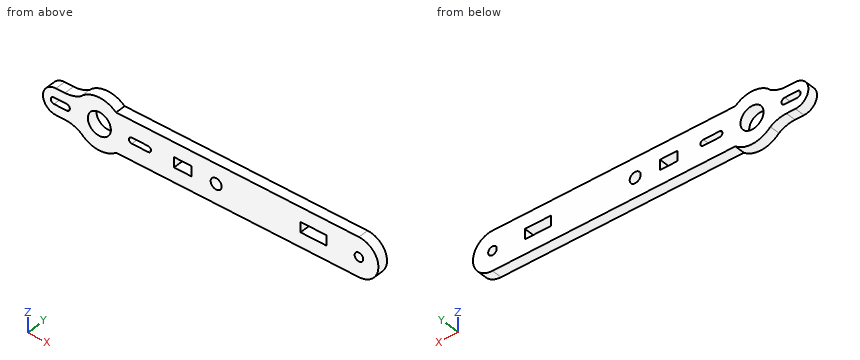
```python
from build123d import *

# Parameters (mm, degrees)
SKETCH1_R           = 1.322622219
SKETCH1_R_2         = 1.7
SKETCH1_R_3         = 3.543581518
SKETCH1_W           = 5.363642664
SKETCH1_H           = 3.09972609
BOSS_EXTRUDE1_DEPTH = 3.175


with BuildPart() as part:
    # Sketch1 → Boss-Extrude1 (new body)
    with BuildSketch(Plane(origin=(0, 0, 0), x_dir=(1, 0, 0), z_dir=(0, 1, 0))):
        with BuildLine():
            Line((-30.420224954, 6.394505262), (44.302185909, 6.390032423))
            ThreePointArc((44.302185909, 6.390032423), (50.304735151, 0.387483181), (44.302185909, -5.61506606))
            Line((44.302185909, -5.61506606), (-30.420308604, -5.61506606))
            ThreePointArc((-30.420308604, -5.61506606), (-36.033562007, -7.500021548), (-41.380965097, -4.957001462))
            ThreePointArc((-41.380965097, -4.957001462), (-43.672708861, -3.953506377), (-46.150888165, -3.610404055))
            Line((-46.150888165, -3.610404055), (-48.909665253, -3.610404055))
            ThreePointArc((-48.909665253, -3.610404055), (-52.90984424, 0.389774933), (-48.909665253, 4.38995392))
            Line((-48.909665253, 4.38995392), (-46.150888165, 4.38995392))
            ThreePointArc((-46.150888165, 4.38995392), (-43.564402624, 4.780712621), (-41.208786399, 5.918109658))
            ThreePointArc((-41.208786399, 5.918109658), (-35.908549497, 8.286044856), (-30.420224954, 6.394505262))
        make_face()
        with Locations(Location((44.302185909, 0.387483181, 0), (0, 0, 270))):
            Circle(SKETCH1_R, mode=Mode.SUBTRACT)
        with Locations(Location((0.383109325, 0.385153592, 0), (0, 0, 270))):
            Circle(SKETCH1_R_2, mode=Mode.SUBTRACT)
        with Locations(Location((-35.559869313, 0.389755399, 0), (0, 0, 270))):
            Circle(SKETCH1_R_3, mode=Mode.SUBTRACT)
        Polygon((34.320012777, 1.885218269), (34.320012777, 1.935143597), (26.334122715, 1.935143597), (26.334122715, 1.885218269), (26.334122715, -1.114852491), (26.334122715, -1.164973144), (34.320012777, -1.164973144), (34.320012777, -1.114852491), align=None, mode=Mode.SUBTRACT)
        with Locations((-9.914943428, 0.385085228)):
            Rectangle(SKETCH1_W, SKETCH1_H, mode=Mode.SUBTRACT)
        with BuildLine():
            Line((-20.582664571, -0.514889121), (-25.573840985, -0.514889121))
            ThreePointArc((-25.573840985, -0.514889121), (-26.473815335, 0.385085229), (-25.573840985, 1.285059578))
            Line((-25.573840985, 1.285059578), (-20.582664571, 1.285059578))
            ThreePointArc((-20.582664571, 1.285059578), (-19.682690221, 0.385085229), (-20.582664571, -0.514889121))
        make_face(mode=Mode.SUBTRACT)
        with BuildLine():
            Line((-49.512218616, 1.385222757), (-45.638080248, 1.385222757))
            ThreePointArc((-45.638080248, 1.385222757), (-44.638040384, 0.385182893), (-45.638080248, -0.614856971))
            Line((-45.638080248, -0.614856971), (-49.512218616, -0.614856971))
            ThreePointArc((-49.512218616, -0.614856971), (-50.51225848, 0.385182893), (-49.512218616, 1.385222757))
        make_face(mode=Mode.SUBTRACT)
    extrude(amount=BOSS_EXTRUDE1_DEPTH)


solid = part.part
```
Verification items for the finished model (mm, model axes). Round coordinates to 2 decimals unless told otherwise and drop trailing zeros. Order: outer loops, then holes, each group sorted by start corner. A loop starts at its lowest first (then second) coordinate and runs counter-clockwise, first axis right, second up. Notation, with made-up numbers: (60.25, -6.5) - (93.25, -6.5) arc R17 cw to (93.25, 25.5) - close; hole circle Ø3 at (-14.5, 27.25). An arc over 180 degrees is marked (long way). Use CSV: the item, a comma, the result in double quotes.
(1) Thickness scan on probe 1 along Z at (x, y) = (-48.5, 2.55); probe 2 along Z at (x, y) = (8.5, 1.6); probe 3 along X at (y, z) = (1.6, 2). Record the ranges inside material, lowest first. Write a range as from..to.
Entries:
probe 1,"-4.39..-1.39, 0.61..3.61"
probe 2,"-6.39..5.62"
probe 3,"-52.12..-38.18, -32.94..49.81"
(2) Section check C-C on x = 33. Record the boundary of the cut face in (y, z) (3 decimals), and give its area (3 significant figures).
Entries:
outline,"(0, -6.391) - (3.175, -6.391) - (3.175, -1.935) - (0, -1.935) - close; (0, 1.165) - (3.175, 1.165) - (3.175, 5.615) - (0, 5.615) - close"
area,"28.3 mm^2"
(3) Section check A-A on x = -9. Record the boundary of the cut face in (y, z) (3 decimals).
Entries:
outline,"(0, -6.393) - (3.175, -6.393) - (3.175, -1.935) - (0, -1.935) - close; (0, 1.165) - (3.175, 1.165) - (3.175, 5.615) - (0, 5.615) - close"
(4) Gauge pin test, flat ends, axial feed: pin 1 Ø3 at (x, z) = (-29.5, -4.5) entering from -Y; pin 2 Ø0.9 at (y, z) = (1, -1) entering from -X; pin 3 Ø1.6 at (x, y) = (30, 1.5) entering from -Z; pin 4 Ø0.8 at (x, y) = (-48, 2) entering from +Z. Record the tip position at first contact, or that the pin passes through.
Entries:
pin 1,"y = 0"
pin 2,"x = -52.91"
pin 3,"z = -6.39"
pin 4,"z = 3.61"
(5) Section check D-D on x = 17. Record the boundary of the cut face in (y, z) (3 decimals).
Entries:
outline,"(0, -6.392) - (3.175, -6.392) - (3.175, 5.615) - (0, 5.615) - close"
(6) Section check B-B on y = 1.3. State how many separate pieces and enclosed holes the cut face has, and give its area (3 significant figures).
Entries:
separate pieces,"1"
enclosed holes,"7"
area,"1,080 mm^2"
